from build123d import *

# Parameters (mm, degrees)
ESQUISSE2_R             = 1.35
BOSS_EXTRU_2_DEPTH      = 6
BOSS_EXTRU_3_START      = -6
ESQUISSE3_R             = 1.35
BOSS_EXTRU_3_DEPTH      = 6
ENL_V_MAT_EXTRU_1_DEPTH = 3


with BuildPart() as part:
    # Esquisse1 → Révolution1 (revolve)
    with BuildSketch(Plane.XY, mode=Mode.PRIVATE) as r_volution1_sk:
        Polygon((-6.05, 0), (-6.05, 4), (-3.85, 4), (-3.25, 4.6), (-3.25, 25.8), (-3.85, 26.4), (-6.05, 26.4), (-6.05, 30.4), (-8, 30.4), (-8, 24.4), (-7, 23.4), (-7, 7), (-8, 6), (-8, 0), align=None)
    revolve(r_volution1_sk.sketch.rotate(Axis((0, 0, 0), (0, 1, 0)), 270), axis=Axis((0, 0, 0), (0, 1, 0)))

    # Esquisse2 → Boss.-Extru.2 (add)
    with BuildSketch(Plane(origin=(0, 0, 0), x_dir=(1, 0, 0), z_dir=(0, 1, 0))):
        with BuildLine():
            Line((-7.878088106, -1.391304348), (-3.939044053, -23.695652174))
            ThreePointArc((-3.939044053, -23.695652174), (0, -27), (3.939044053, -23.695652174))
            Line((3.939044053, -23.695652174), (7.878088106, -1.391304348))
            ThreePointArc((7.878088106, -1.391304348), (0, -8), (-7.878088106, -1.391304348))
        make_face()
        with Locations(Location((0, -23, 0), (0, 0, 90))):
            Circle(ESQUISSE2_R, mode=Mode.SUBTRACT)
    extrude(amount=BOSS_EXTRU_2_DEPTH)

    # Esquisse3 → Boss.-Extru.3 (add)
    with BuildSketch(Plane(origin=(0, 30.4, 0), x_dir=(1, 0, 0), z_dir=(0, 1, 0)).offset(BOSS_EXTRU_3_START)):
        with BuildLine():
            Line((21.761904762, 3.926767262), (1.523809524, 7.853534525))
            ThreePointArc((1.523809524, 7.853534525), (8, 0), (1.523809524, -7.853534525))
            Line((1.523809524, -7.853534525), (21.761904762, -3.926767262))
            ThreePointArc((21.761904762, -3.926767262), (25, 0), (21.761904762, 3.926767262))
        make_face()
        with Locations(Location((21, 0, 0), (0, 0, 270))):
            Circle(ESQUISSE3_R, mode=Mode.SUBTRACT)
    extrude(amount=BOSS_EXTRU_3_DEPTH)

    # Esquisse4 → Enlèv. mat.-Extru.1 (cut)
    with BuildSketch(Plane.XZ.offset(-24.4)):
        Polygon((21, -3.175426481), (23.75, -1.58771324), (23.75, 1.58771324), (21, 3.175426481), (18.25, 1.58771324), (18.25, -1.58771324), align=None)
    extrude(amount=-ENL_V_MAT_EXTRU_1_DEPTH, mode=Mode.SUBTRACT)


solid = part.part
Model file for the job. Use its own axes, mm. A direction names the side the tool comes from. Give positions to 0.01 mm unless a question says otherwise; leave off trailing zeros. Order: outer loops, then holes, each group sorted by start corner. A loop starts at its lowest first (then second) coordinate and runs counter-clockwise, first axis right, second up. Notation, with made-up numbers: (63.25, -25.5) - (110.25, -25.5) arc R21 cw to (110.25, -11.5) - close; hole circle Ø2 at (-33.75, 42). An arc over 180 degrees is marked (long way). One line per item, written item: value.
Item 1: Slice it at B-B (y = 19). List the corners of the cut face in (x, z).
Response values:
outline: circle Ø14 at (0, 0); hole circle Ø6.5 at (0, 0)
Item 2: Slice it at A-A (z = 23). List the corners of the cut face in (x, y), then the cut area to 3 significant figures.
Response values:
outline: (-4.06, 0) - (-1.35, 0) - (-1.35, 6) - (-4.06, 6) - close; (1.35, 0) - (4.06, 0) - (4.06, 6) - (1.35, 6) - close
area: 32.5 mm2
Item 3: Pin check, flat tips, straight feed: pin 1 Ø4 at (x, y) = (3, 13) entering from +Z; pin 2 Ø6 at (x, z) = (21, 1.5) entering from -Y; pin 3 Ø6 at (x, z) = (0, 0) entering from -Y; pin 4 Ø9.5 at (x, z) = (1, 0) entering from +Y. Stop position of each tip, or through.
Response values:
pin 1: z = 6.93
pin 2: y = 24.4
pin 3: through
pin 4: y = 26.4
Item 4: Tool access for faces 5 (the flat face through (5.88, 2.96, 12.7)), 6 (the flat face through (11.501, 27.358, 5.918)), 7 (the flat face through (22.394, 25.879, 2.37)), 8 (the cylindrical face through (6.834, 15.085, 1.517)): list every direction of +Z, -Z, +X, -X, +Y, -Y with a clear straight run to the whole face (end or side of a thin tool).
Response values:
face 5: +Z, +X, -Y
face 6: +Z, +X, +Y
face 7: -Y
face 8: none
Item 5: Wall check: line 1 (X direction, y = 28.55, z = 0); line 2 (X direction, y = 1.8, z = 0); line 3 (Y direction, x = 16, z = -2). Give the ranges that are in metal, low to high.
Response values:
line 1: -8 to -6.05, 6.05 to 19.65, 22.35 to 25
line 2: -8 to -6.05, 6.05 to 8
line 3: 24.4 to 30.4
Item 6: Slice it at D-D (z = 17). List the corners of the cut face in (x, y).
Response values:
outline: (-5.12, 0) - (5.12, 0) - (5.12, 6) - (-5.12, 6) - close
Item 7: Slice it at C-C (z = 0). Give the number of separate pieces and of enclosed holes in the cut face, then the cut area to 3 significant figures.
Response values:
separate pieces: 3
enclosed holes: 0
area: 286 mm2
Item 8: Two-plate mould, pull along Z, no slides. Class faces 1 (the flat face through (19.64, 25.88, 2.39)), 2 (the cylindrical face through (-8, 27, 0)), 3 (the cylindrical face through (-1.82, 2.03, -5.77)), 4 (the flat face through (0, 6, 14)): released by +Z, released by -Z, zero draft, split by the parting line, or undercut.
Response values:
face 1: undercut
face 2: split by the parting line
face 3: undercut
face 4: zero draft
